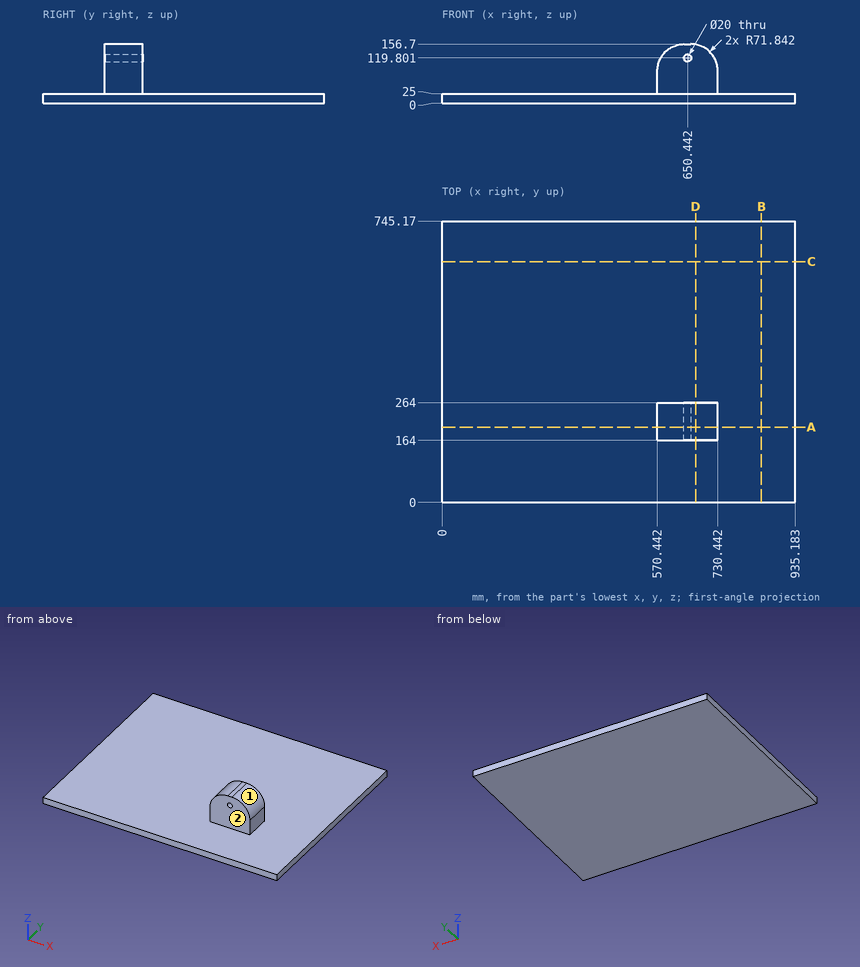
The figure shows three views and two pictorial views of one solid part (mm, origin at its lowest corner). Answer the questions. A direction names the side the tool comes from. Round coordinates to 2 decimals unless told otherwise and drop trailing zeros. Write each loop counter-clockwise with the first axis right and the second up, starting at its lowest first coordinate (ties: lowest second). Pieces come first, ordered by that corner, then holes. Notation, with made-up numbers: (62, -40) -> (88, -40) arc R15 cw to (88, -31) -> close; hole circle Ø5 at (77.5, 86). An arc over 180 degrees is marked (long way). Write each question's results on one line, items separated by ' | '.
Q1. Which of the six approach directions +Z, -Z, +X, -X, +Y, -Y give full straight-line access (tool end or side, diameter ignored) to the marked faces 1 and 2?
Data:
face 1: +Z, +X, +Y, -Y | face 2: +Z, +X, -X, -Y
Q2. Flat-ended cylindrical pins translate along their axes: P1, Ø1, axis at x = 365, y = 219, coming from the -Z side; P2, Ø8, axis at x = 675.5, z = 139.5, coming from the +Y side; P3, Ø10, axis at x = 104.5, y = 458, coming from the +Z side. Find the tip coordinate at first contact, or state that the pin passes through.
Data:
P1: z = 0 | P2: y = 264 | P3: z = 25
Q3. Section B-B, the plane x = 846 is taken. Write down the section's boundary in (y, z), then the cut area to 3 significant figures.
Data:
outline: (0, 0) -> (745.17, 0) -> (745.17, 25) -> (0, 25) -> close | area: 18,600 mm^2
Q4. Section C-C, the plane y = 637.5 is taken. Write down the section's boundary in (x, z).
Data:
outline: (0, 0) -> (935.18, 0) -> (935.18, 25) -> (0, 25) -> close
Q5. Section A-A, the plane y = 199 is taken. Write down the section's boundary in (x, z) (1 decimal).
Data:
outline: (0, 0) -> (935.2, 0) -> (935.2, 25) -> (730.4, 25) -> (730.4, 84.9) arc R71.8 ccw to (658.6, 156.7) -> (642.3, 156.7) arc R71.8 ccw to (570.4, 84.9) -> (570.4, 25) -> (0, 25) -> close; hole circle Ø20 at (650.4, 119.8)
Q6. Section D-D, the plane x = 671.5 is taken. Write down the section's boundary in (y, z).
Data:
outline: (0, 0) -> (745.17, 0) -> (745.17, 25) -> (264, 25) -> (264, 155.53) -> (164, 155.53) -> (164, 25) -> (0, 25) -> close
Q7. Straight lines are drawn through the part: line 1 along Z through (x, y) = (123.5, 631.5); line 2 along X through (y, z) = (235, 50); line 3 along Y through (x, z) = (679, 43). For each, find the intervals that lie inside material, in ascending order. Write a range as [from, to].
Data:
line 1: [0, 25] | line 2: [570.44, 730.44] | line 3: [164, 264]
